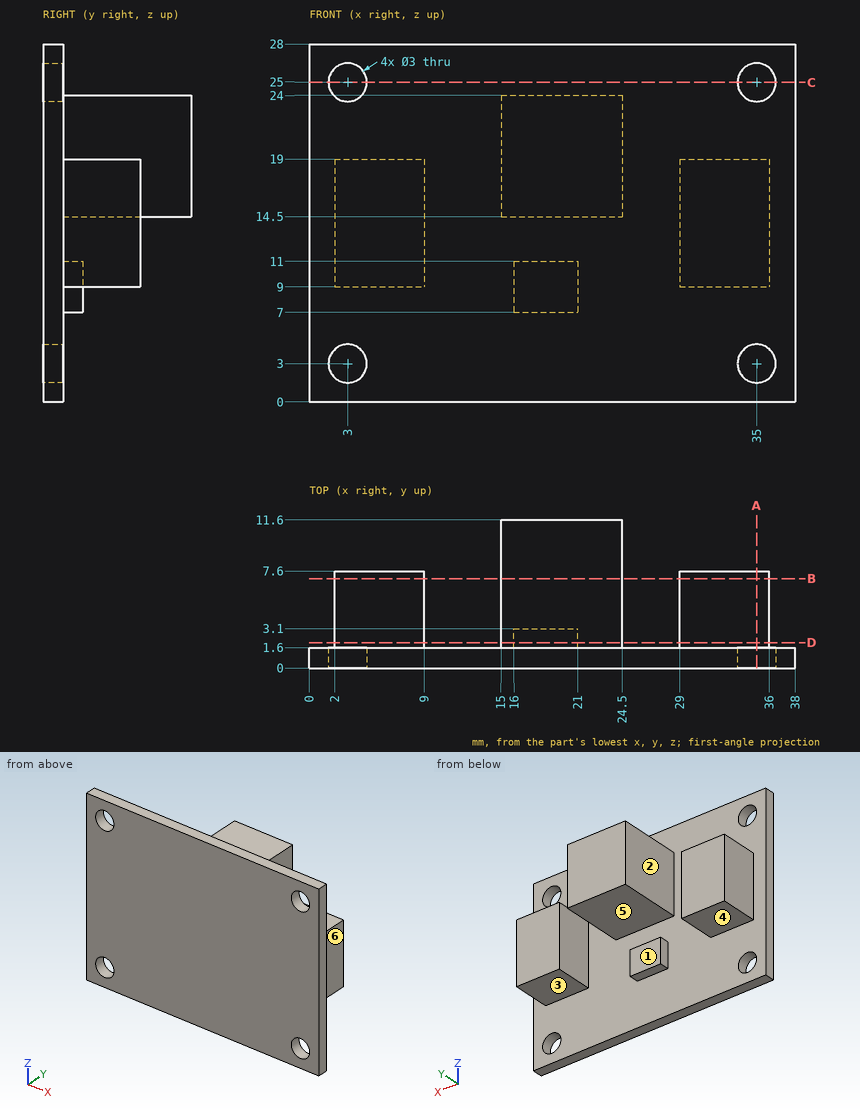
For this review, use the dimensioned drawing (mm, ordinates from the lowest corner) and the shaded views. A direction names the side the tool comes from. Round coordinates to 2 decimals unless told otherwise and drop trailing zeros. Write each loop counter-clockwise with the first axis right and the second up, starting at its lowest first coordinate (ties: lowest second). Pieces come first, ordered by that corner, then holes. Notation, with made-up numbers: M 8,-39 L 32,-39 A11 cw 32,-29 Z; hole C -34,42.25 d7. An arc over 180 degrees is marked long. Use CSV: the item, a comma, the result in double quotes. Start each with the question number.
(1) Clearance check with flat-ended pins moving along their axes: P1, Ø3, axis at y = 9.5, z = 22, coming from the +X side; P2, Ø5.5, axis at x = 33.5, z = 14, coming from the +Y side; P3, Ø5, axis at x = 18.5, y = 6.5, coming from the -Z side. State where each tip first meets the part, or that it passes through.
(2) We need section C-C, the plane z = 25. State the section outline as (x, y) points, then the cut area to 3 significant figures.
(3) The part is to be moulded in two halves that separate along X. For the marked faces 4, 5 and 6, say which applies: +X half, -X half, draft (parallel to the pull), parting line (faces both ways), or undercut.
(4) We need section B-B, the plane y = 7. State the section outline as (x, z) points.
(5) We need section A-A, the plane x = 35. State the section outline as (y, z) points, then the cut area to 3 significant figures.
(6) Tool access review of the marked faces 1, 2 and 3: name each direction out of +Z, -Z, +X, -X, +Y, -Y from which nothing blocks a thin tool from reaching the whole face with its end or side.
(7) We need section D-D, the plane y = 2. State the section outline as (x, z) points.
(8) For line 1 along X through (y, z) = (0.85, 25); line 2 along Z through (x, y) = (35, 1.1); line 3 along Z through (x, y) = (18, 11.25), list the stretches that pass through material, from the lowest coordinate up.
Findings:
1,P1,"x = 24.5"
1,P2,"y = 7.6"
1,P3,"z = 14.5"
2,outline,"M 0,0 L 1.5,0 L 1.5,1.6 L 0,1.6 Z; M 4.5,0 L 33.5,0 L 33.5,1.6 L 4.5,1.6 Z; M 36.5,0 L 38,0 L 38,1.6 L 36.5,1.6 Z"
2,area,"51.2 mm^2"
3,face 4,"draft"
3,face 5,"undercut"
3,face 6,"+X half"
4,outline,"M 2,9 L 9,9 L 9,19 L 2,19 Z; M 15,14.5 L 24.5,14.5 L 24.5,24 L 15,24 Z; M 29,9 L 36,9 L 36,19 L 29,19 Z"
5,outline,"M 0,0 L 1.6,0 L 1.6,1.5 L 0,1.5 Z; M 0,4.5 L 1.6,4.5 L 1.6,9 L 7.6,9 L 7.6,19 L 1.6,19 L 1.6,23.5 L 0,23.5 Z; M 0,26.5 L 1.6,26.5 L 1.6,28 L 0,28 Z"
5,area,"95.2 mm^2"
6,face 1,"-Z, +Y"
6,face 2,"+Z, -Z, +Y"
6,face 3,"-Z, +X, +Y"
7,outline,"M 2,9 L 9,9 L 9,19 L 2,19 Z; M 15,14.5 L 24.5,14.5 L 24.5,24 L 15,24 Z; M 16,7 L 21,7 L 21,11 L 16,11 Z; M 29,9 L 36,9 L 36,19 L 29,19 Z"
8,line 1,"0 to 1.5, 4.5 to 33.5, 36.5 to 38"
8,line 2,"0 to 1.5, 4.5 to 23.5, 26.5 to 28"
8,line 3,"14.5 to 24"
